from build123d import *

# Parameters (mm, degrees)
F0_R     = 13.5
F0_R_2   = 10
F1_DEPTH = 1
F0_R_3   = 17.5
F2_DEPTH = 2
F0_R_4   = 20
F3_DEPTH = 7
F5_START = 4
F4_R     = 20
F4_R_2   = 16
F5_DEPTH = 3
F6_R     = 1


with BuildPart() as f1:
    # F0 (on Top) → F1 (new body)
    with BuildSketch(Plane.XY):
        Circle(F0_R)
        Circle(F0_R_2, mode=Mode.SUBTRACT)
    extrude(amount=F1_DEPTH)

    # F0 (on Top) → F2 (join)
    with BuildSketch(Plane.XY):
        Circle(F0_R_3)
        Circle(F0_R, mode=Mode.SUBTRACT)
    extrude(amount=F2_DEPTH)

    # F0 (on Top) → F3 (join)
    with BuildSketch(Plane.XY):
        Circle(F0_R_4)
        Circle(F0_R_3, mode=Mode.SUBTRACT)
    extrude(amount=F3_DEPTH)

    # F4 (on Top) → F5 (join)
    with BuildSketch(Plane.XY.offset(F5_START)):
        Circle(F4_R)
        Circle(F4_R_2, mode=Mode.SUBTRACT)
    extrude(amount=F5_DEPTH)

    # F6
    f6_edges = [f1.edges().sort_by_distance(p)[0] for p in [
        (-16, 0, 4),
    ]]
    fillet(f6_edges, radius=F6_R)


solid = f1.part
The model under review builds one solid part; all positions refer to its coordinate system, in mm. A direction names the side the tool comes from. Give positions to 0.01 mm unless a question says otherwise; leave off trailing zeros. Order: outer loops, then holes, each group sorted by start corner. A loop starts at its lowest first (then second) coordinate and runs counter-clockwise, first axis right, second up. Notation, with made-up numbers: (9, 36.5) -> (24, 36.5) arc R5 ccw to (24, 44.5) -> close; hole circle Ø2 at (61.25, 11.5). An arc over 180 degrees is marked (long way). Write item = value, one per line. Start each with the question number.
(1) Take a section at A-A (y = 0). Write out the cut boundary in (x, z), plus the area to 3 significant figures.
(2) Tool access review of faces 5 (the flat face through (-3, 17, 4)), 6 (the cylindrical face through (-2.93, -13.18, 1.49)), 7 (the flat face through (-5, 9, 0)): name each direction out of +Z, -Z, +X, -X, +Y, -Y from which nothing blocks a thin tool from reaching the whole face with its end or side.
(3) For L1, parallel to Y at x = 0, z = 6.65; L2, parallel to Z at x = 11.5, y = -7.5; L3, parallel to Y at x = 14.5, z = 5.25, list the stretches that pass through material, from the lowest coordinate up. Write a range as from..to.
(4) For pin 1 Ø3 at (x, z) = (7.5, 3.5) entering from +Y; pin 2 Ø3 at (y, z) = (7.5, 4.5) entering from -X; pin 3 Ø19 at (x, y) = (0, 0) entering from -Z; pin 4 Ø1.5 at (y, z) = (12, 3.5) entering from -X, all flat-tipped, find the tip position at first contact; note any pin that passes through.
(5) Draft analysis for pull direction X (two halves, no side actions). For faces 1 (the flat face through (9, -10.3, 2)), 2 (the flat face through (-8.98, 13.43, 7)), 3 (the cylindrical face through (-4.336, -19.524, 3.451)), 4 (the flat face through (-9, -5, 1)), state which applies: +X half, -X half, draft (parallel to the pull), parting line (faces both ways), or undercut.
(6) Take a section at C-C (z = 6). Write out the cut boundary in (x, y), plus the area to 3 significant figures.
Returned:
q1.outline = (-20, 0) -> (-10, 0) -> (-10, 1) -> (-13.5, 1) -> (-13.5, 2) -> (-17.5, 2) -> (-17.5, 4) -> (-17, 4) arc R1 ccw to (-16, 5) -> (-16, 7) -> (-20, 7) -> close; (10, 0) -> (20, 0) -> (20, 7) -> (16, 7) -> (16, 5) arc R1 ccw to (17, 4) -> (17.5, 4) -> (17.5, 2) -> (13.5, 2) -> (13.5, 1) -> (10, 1) -> close
q1.area = 66.6 mm²
q2.face_5 = none
q2.face_6 = +Z
q2.face_7 = -Z, +X, -X, +Y, -Y
q3.L1 = -20..-16, 16..20
q3.L2 = 0..2
q3.L3 = -13.77..-6.76, 6.76..13.77
q4.pin_1 = 19.08
q4.pin_2 = -19.08
q4.pin_3 = through
q4.pin_4 = -16.54
q5.face_1 = undercut
q5.face_2 = draft
q5.face_3 = parting line
q5.face_4 = undercut
q6.outline = circle Ø40 at (0, 0); hole circle Ø32 at (0, 0)
q6.area = 452 mm²
